Input: dimensioned drawing with shaded views. Units: mm. Origin: part minimum x, y, z. A direction names the side the tool comes from. Give positions to 0.01 mm unless a question says otherwise; leave off trailing zeros. Loops run counter-clockwise (first coordinate to the right, second up) from the corner with the lowest first, then second, coordinate; pieces in that order, holes last. Notation, with made-up numbers: (-28, 71.25) -> (25, 71.25) arc R14 cw to (25, 86.25) -> close; hole circle Ø2 at (-13.75, 7.25). An arc over 180 degrees is marked (long way). One line per question, with ' | ' between items. Start each with the question number.
Item 1: Section D-D on y = 37.5. Return loops of the section in (x, z), then the cut area to 3 significant figures.
Item 2: Section A-A on y = 5. Return loops of the section in (x, z).
Item 3: Section B-B on z = 10.25. Return loops of the section in (x, y).
Item 4: Pin query (flat end, axial travel): P1, Ø3, axis at x = 26.5, z = 11, coming from the +Y side; P2, Ø8, axis at x = 21.5, y = 14, coming from the +Z side. Return the tip coordinate at first contact, or that it passes through.
Item 5: Set-up query: the marked faces 1 and 2. Return all of +Z, -Z, +X, -X, +Y, -Y with unobstructed straight access to the full face (end or side cutting, diameter ignored); none if empty.
Item 6: Section C-C on x = 31. Return loops of the section in (y, z).
Item 7: Material intervals for line 1 along Z through (x, y) = (28, 13.5); line 2 along Y through (x, z) = (38.5, 3.25); line 3 along Y through (x, z) = (13.5, 1.75), sorted ascending. Write a range as [from, to].
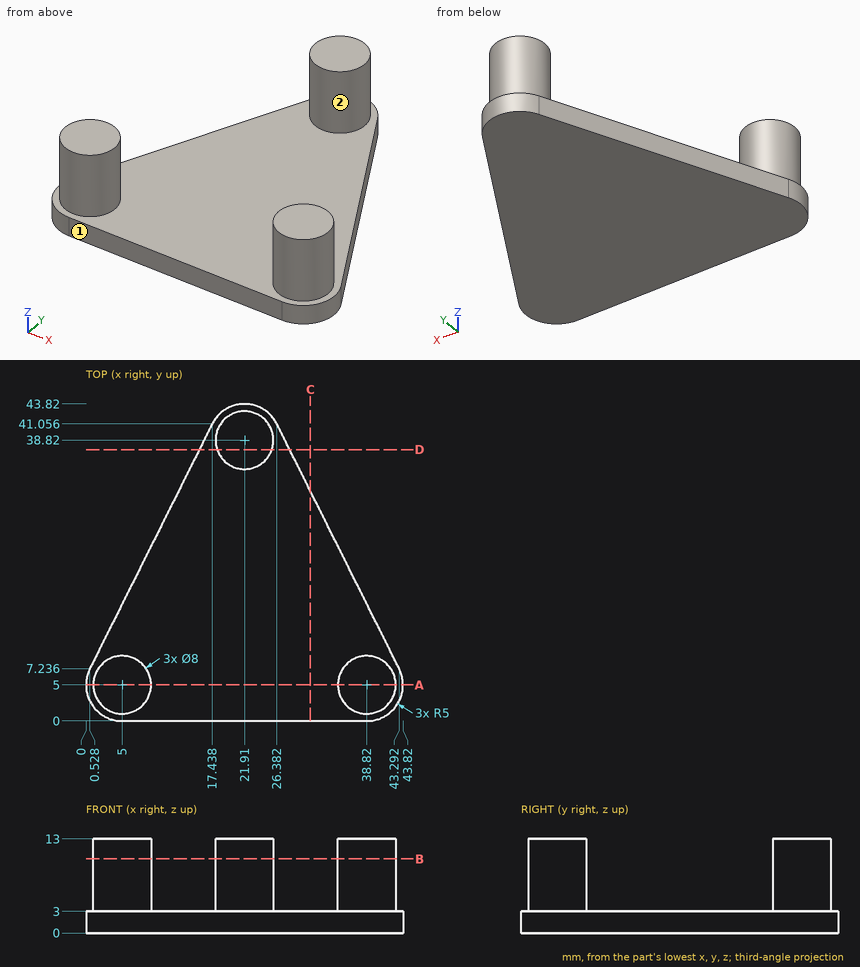
Result sheet:
1) outline: (15.66, 0) -> (28.16, 0) -> (28.16, 3) -> (25.69, 3) -> (25.69, 13) -> (18.13, 13) -> (18.13, 3) -> (15.66, 3) -> close | area: 113 mm²
2) outline: (0, 0) -> (43.82, 0) -> (43.82, 3) -> (42.82, 3) -> (42.82, 13) -> (34.82, 13) -> (34.82, 3) -> (9, 3) -> (9, 13) -> (1, 13) -> (1, 3) -> (0, 3) -> close
3) outline: circle Ø8 at (5, 5); circle Ø8 at (21.91, 38.82); circle Ø8 at (38.82, 5)
4) P1: stops at y = 41.36 | P2: stops at z = 3
5) face 1: +Z, -Z, +X, -X, -Y | face 2: +Z
6) outline: (0, 0) -> (31.82, 0) -> (31.82, 3) -> (0, 3) -> close
7) line 1: z = [0, 3] | line 2: y = [1.01, 8.99] | line 3: y = [0, 33.18]
